Part print with two shaded views. Sizes in mm from the minimum x, y, z corner. A direction names the side the tool comes from. Give positions to 0.01 mm unless a question says otherwise; leave off trailing zeros. Loops run counter-clockwise (first coordinate to the right, second up) from the corner with the lowest first, then second, coordinate; pieces in that order, holes last. Notation, with made-up numbers: M -13.75,-16 L 17.25,-16 A22 cw 17.25,16 Z; hole C 1.5,12 d4. An arc over 180 degrees is marked long. Answer in a Markdown table with one row per item.
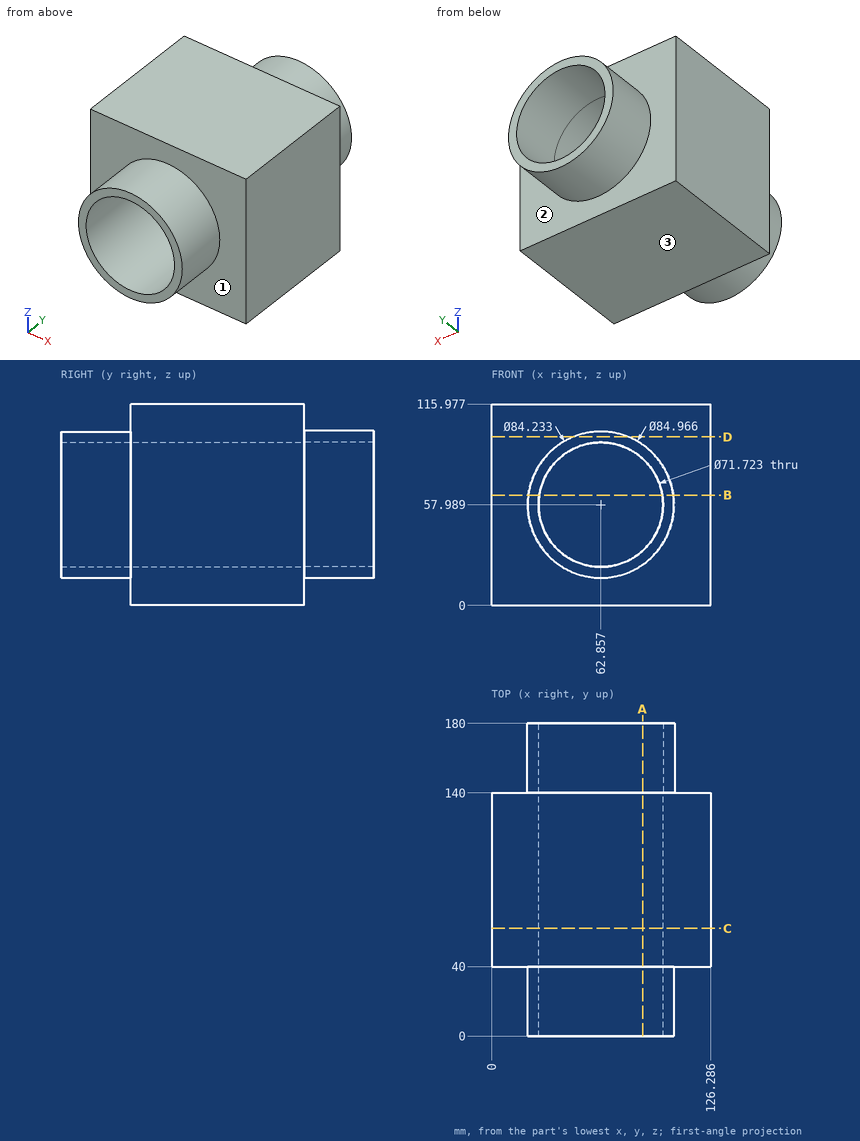
Q1. Drop flat-ended pins along their axis: pin 1 (1 mm diameter, centred on x = 106, z = 98.5, fed in from -Y); pin 2 (1.5 mm diameter, centred on x = 53.5, y = 26.5, fed in from +Z). Give the stop position or say it passes through.
Reported:
| item | result |
|---|---|
| pin 1 | y = 40 |
| pin 2 | z = 99.22 |
Q2. Probe probe 1 along X at (y, z) = (78, 57.5) (1 decimal); probe 2 along Z at (x, y) = (88.5, 126) (1 decimal); probe 3 along Z at (x, y) = (76.5, 67) (1 decimal). List the from-to ranges inside material, lowest first.
Reported:
| item | result |
|---|---|
| probe 1 | 0 to 27, 98.7 to 126.3 |
| probe 2 | 0 to 32.9, 83.1 to 116 |
| probe 3 | 0 to 24.8, 91.2 to 116 |
Q3. Saw through at C-C (y = 62). Give the cut face in (x, z).
Reported:
| item | result |
|---|---|
| outline | M 0,0 L 126.29,0 L 126.29,115.98 L 0,115.98 Z; hole C 62.86,57.99 d71.72 |
Q4. Saw through at B-B (z = 63.5). Give the cut face in (x, y).
Reported:
| item | result |
|---|---|
| outline | M 0,40 L 21.1,40 L 21.1,0 L 27.42,0 L 27.42,180 L 20.73,180 L 20.73,140 L 0,140 Z; M 98.29,0 L 104.61,0 L 104.61,40 L 126.29,40 L 126.29,140 L 104.98,140 L 104.98,180 L 98.29,180 Z |
Q5. Saw through at D-D (z = 97). Give the cut face in (x, y) (1 decimal).
Reported:
| item | result |
|---|---|
| outline | M 0,40 L 47,40 L 47,0 L 78.7,0 L 78.7,40 L 126.3,40 L 126.3,140 L 79.7,140 L 79.7,180 L 46,180 L 46,140 L 0,140 Z |
Q6. Saw through at A-A (x = 87). Give the cut face in (y, z) (1 decimal), and give its area (3 significant figures).
Reported:
| item | result |
|---|---|
| outline | M 0,23.5 L 40,23.5 L 40,0 L 140,0 L 140,23 L 180,23 L 180,31.5 L 0,31.5 Z; M 0,84.5 L 180,84.5 L 180,92.9 L 140,92.9 L 140,116 L 40,116 L 40,92.5 L 0,92.5 Z |
| area | 7,610 mm² |
Q7. 3-axis set-ups, long thin cutter, end or side, ignore diameter. For the marked faces 1, 2 and 3: which of +Z, -Z, +X, -X, +Y, -Y reach the whole face in a straight line?
Reported:
| item | result |
|---|---|
| face 1 | -Y |
| face 2 | +Y |
| face 3 | -Z, +X, -X, +Y, -Y |
